The model under review builds one solid part; all positions refer to its coordinate system, in mm. A direction names the side the tool comes from. Round coordinates to 2 decimals unless told otherwise and drop trailing zeros. Order: outer loops, then holes, each group sorted by start corner. A loop starts at its lowest first (then second) coordinate and runs counter-clockwise, first axis right, second up. Notation, with made-up numbers: (86, -30.5) - (107, -30.5) arc R29 cw to (107, 1.5) - close; hole circle Ø4 at (5.5, 70). An arc over 180 degrees is marked (long way). One line per question, with ' | ' between items. Start each with the question number.
Item 1: Insertion check: pin 1 Ø2.5 at (y, z) = (-11.5, 6) entering from -X; pin 2 Ø4 at (x, y) = (-12.5, 1.5) entering from +Z; pin 3 Ø9 at (y, z) = (9.5, 4) entering from +X. Each pin has a flat end and moves straight along its axis. Give the tip position at first contact, or say it passes through.
Item 2: Add section B-B on z = 6. State the section outline as (x, y) points, and give its area (3 significant figures).
Item 3: For L1, parallel to X at y = 0, z = 21.5; L2, parallel to Y at x = 1.25, z = 19, list the stretches that pass through material, from the lowest coordinate up. Write a range as [from, to].
Item 4: Add section D-D on x = 0. State the section outline as (y, z) points, and give its area (3 significant figures).
Item 5: Add section A-A on y = 0. State the section outline as (x, z) points, and give its area (4 significant figures).
Item 6: Add section C-C on x = -5.25. State the section outline as (y, z) points.
Item 7: Tool access review of faces 1 (the face through (-10, -4, 5)), 2 (the face through (10, 4, 5)), 3 (the face through (10, -4, 5)), 4 (the face through (-10, 4, 5)): name each direction out of +Z, -Z, +X, -X, +Y, -Y from which nothing blocks a thin tool from reaching the whole face with its end or side.
from build123d import *

# Parameters (mm, degrees)
ESBO_O1_R                = 15
RESSALTO_EXTRUS_O1_DEPTH = 10
ESBO_O2_R                = 7.5
RESSALTO_EXTRUS_O2_DEPTH = 15
ESBO_O3_R                = 4
CORTE_EXTRUS_O1_DEPTH    = 15
CORTE_EXTRUS_O2_DEPTH    = 20
ESBO_O5_R                = 1.5
CORTE_EXTRUS_O3_DEPTH    = 20


with BuildPart() as part:
    # Esboço1 → Ressalto-extrusão1 (new body)
    with BuildSketch(Plane.XY):
        Circle(ESBO_O1_R)
    extrude(amount=RESSALTO_EXTRUS_O1_DEPTH)

    # Esboço2 → Ressalto-extrusão2 (add)
    with BuildSketch(Plane.XY.offset(10)):
        Circle(ESBO_O2_R)
    extrude(amount=RESSALTO_EXTRUS_O2_DEPTH)

    # Esboço3 → Corte-extrusão1 (cut)
    with BuildSketch(Plane.XY.offset(25)):
        Circle(ESBO_O3_R)
    extrude(amount=-CORTE_EXTRUS_O1_DEPTH, mode=Mode.SUBTRACT)

    # Esboço4 → Corte-extrusão2 (cut)
    with BuildSketch(Plane(origin=(0, 0, 0), x_dir=(-1, 0, 0), z_dir=(0, 0, -1))):
        with BuildLine():
            Line((-4, 6.34428877), (-4, 14.456832295))
            ThreePointArc((-4, 14.456832295), (-10.606601718, 10.606601718), (-14.456832295, 4))
            Line((-14.456832295, 4), (-6.34428877, 4))
            ThreePointArc((-6.34428877, 4), (-5.303300859, 5.303300859), (-4, 6.34428877))
        make_face()
        with BuildLine():
            Line((4, -14.456832295), (4, -6.34428877))
            ThreePointArc((4, -6.34428877), (5.303300859, -5.303300859), (6.34428877, -4))
            Line((6.34428877, -4), (14.456832295, -4))
            ThreePointArc((14.456832295, -4), (10.606601718, -10.606601718), (4, -14.456832295))
        make_face()
        with BuildLine():
            Line((-4, -14.456832295), (-4, -6.34428877))
            ThreePointArc((-4, -6.34428877), (-5.303300859, -5.303300859), (-6.34428877, -4))
            Line((-6.34428877, -4), (-14.456832295, -4))
            ThreePointArc((-14.456832295, -4), (-10.606601718, -10.606601718), (-4, -14.456832295))
        make_face()
        with BuildLine():
            Line((14.456832295, 4), (6.34428877, 4))
            ThreePointArc((6.34428877, 4), (5.303300859, 5.303300859), (4, 6.34428877))
            Line((4, 6.34428877), (4, 14.456832295))
            ThreePointArc((4, 14.456832295), (10.606601718, 10.606601718), (14.456832295, 4))
        make_face()
    extrude(amount=-CORTE_EXTRUS_O2_DEPTH, mode=Mode.SUBTRACT)

    # Esboço5 → Corte-extrusão3 (cut)
    with BuildSketch(Plane(origin=(0, 0, 0), x_dir=(0, 0, -1), z_dir=(1, 0, 0))):
        with Locations((-13.004040431, 0)):
            Circle(ESBO_O5_R)
    extrude(amount=-CORTE_EXTRUS_O3_DEPTH, mode=Mode.SUBTRACT)


solid = part.part
Determined:
1) pin 1: x = -4 | pin 2: z = 10 | pin 3: x = 5.59
2) outline: (-14.46, -4) - (-6.34, -4) arc R7.5 ccw to (-4, -6.34) - (-4, -14.46) arc R15 ccw to (4, -14.46) - (4, -6.34) arc R7.5 ccw to (6.34, -4) - (14.46, -4) arc R15 ccw to (14.46, 4) - (6.34, 4) arc R7.5 ccw to (4, 6.34) - (4, 14.46) arc R15 ccw to (-4, 14.46) - (-4, 6.34) arc R7.5 ccw to (-6.34, 4) - (-14.46, 4) arc R15 ccw to start | area: 423 mm2
3) L1: [-7.5, -4], [4, 7.5] | L2: [-7.4, -3.8], [3.8, 7.4]
4) outline: (-15, 0) - (15, 0) - (15, 10) - (7.5, 10) - (7.5, 25) - (4, 25) - (4, 10) - (-4, 10) - (-4, 25) - (-7.5, 25) - (-7.5, 10) - (-15, 10) - close | area: 405 mm2
5) outline: (-15, 0) - (15, 0) - (15, 10) - (7.5, 10) - (7.5, 25) - (4, 25) - (4, 10) - (-4, 10) - (-4, 11.5) - (-7.5, 11.5) - (-7.5, 10) - (-15, 10) - close; (-7.5, 14.5) - (-4, 14.5) - (-4, 25) - (-7.5, 25) - close | area: 394.5 mm2
6) outline: (-5.36, 0) - (5.36, 0) - (5.36, 25) - (-5.36, 25) - close; hole circle Ø3 at (0, 13)
7) face 1: +Z, -Z, -X, -Y | face 2: +Z, -Z, +X, +Y | face 3: +Z, -Z, +X, -Y | face 4: +Z, -Z, -X, +Y
